Source: three-view drawing plus pictorial views. Frame: mm from the lowest corner of the part. Give positions to 0.01 mm unless a question says otherwise; leave off trailing zeros. Write each loop counter-clockwise with the first axis right and the second up, starting at its lowest first coordinate (ties: lowest second). Pieces come first, ordered by that corner, then holes.
Q1. Cut plane A-A on y = 1.4. Count the separate pieces of the cut face and the enclosed holes in it, plus the area to 3 significant figures.
Q2. Line query: L1, parallel to Z at x = 138.6, y = 1; L2, parallel to Z at x = 272.14, y = 3.25; L3, parallel to X at y = 2.45, z = 137.5. Output: solid intervals per line, ascending.
Q3. Cut plane B-B on z = 67. Return the cut outline in (x, y).
Q4. Cut plane C-C on x = 223. Return the cut outline in (y, z), plus the area to 3 significant figures.
Q5. Pin query (flat end, axial travel): pin 1 (1.8 mm diameter, centred on x = 138.6, z = 282.14, fed in from -Y); pin 2 (1.5 mm diameter, centred on y = 4, z = 225, fed in from -X); pin 3 (1 mm diameter, centred on x = 226.5, y = 4, fed in from -Z). Return the tip coordinate at first contact, or that it passes through.
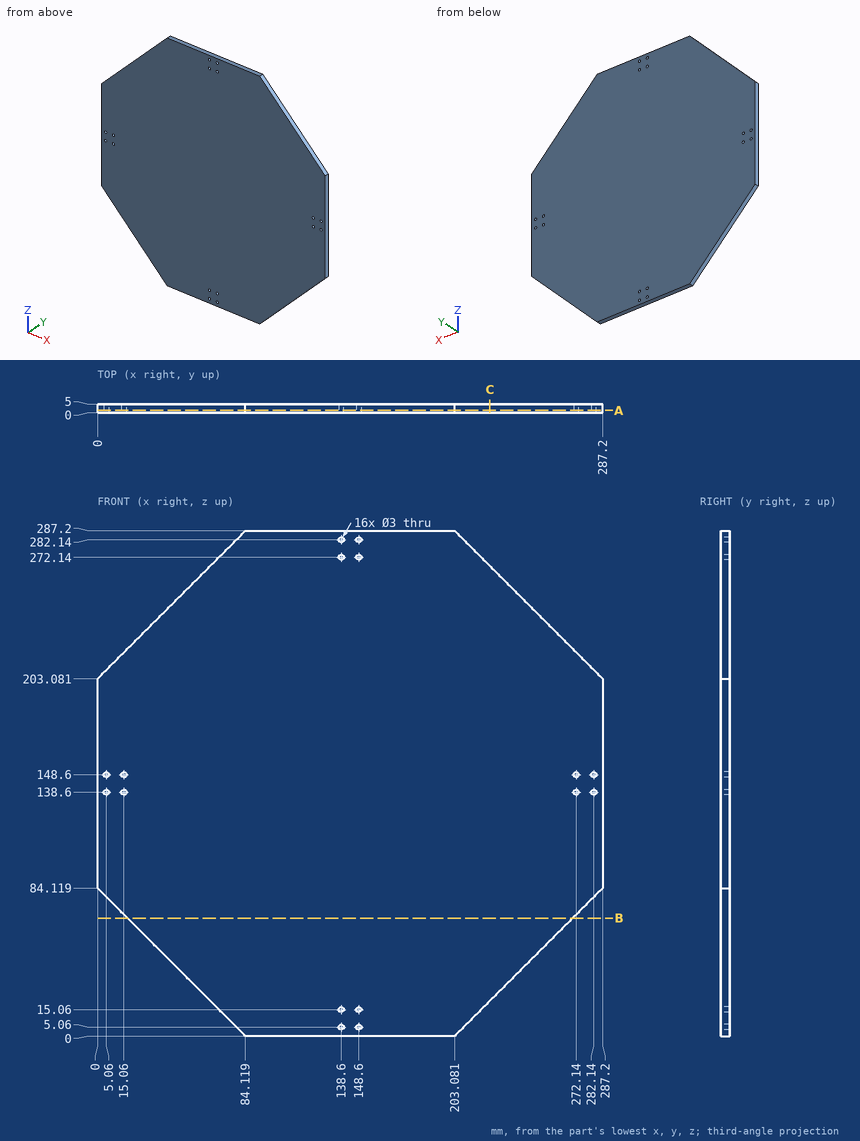
Data:
1. separate pieces: 1
1. enclosed holes: 16
1. area: 68,200 mm2
2. L1: z = 0 to 3.56, 6.56 to 13.56, 16.56 to 270.64, 273.64 to 280.64, 283.64 to 287.2
2. L2: z = 69.06 to 137.1, 140.1 to 147.1, 150.1 to 218.14
2. L3: x = 0 to 4.04, 6.08 to 14.04, 16.08 to 271.12, 273.16 to 281.12, 283.16 to 287.2
3. outline: (17.12, 0) - (270.08, 0) - (270.08, 5) - (17.12, 5) - close
4. outline: (0, 19.92) - (5, 19.92) - (5, 267.28) - (0, 267.28) - close
4. area: 1,240 mm2
5. pin 1: passes through
5. pin 2: stops at x = 21.17
5. pin 3: stops at z = 22.92
